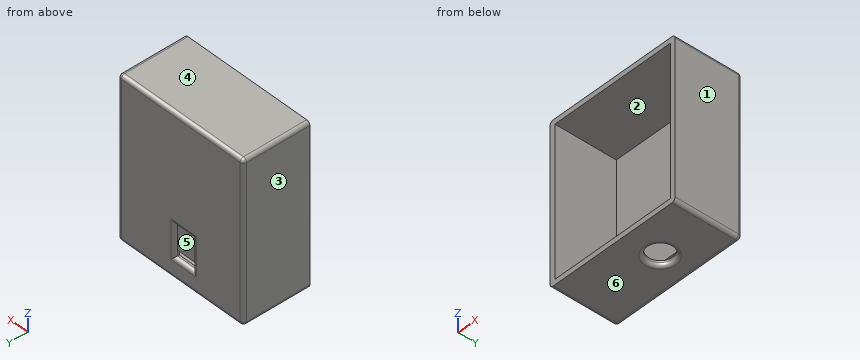
Autodesk Inventor part; units mm, degrees
ref_plane "YZ Plane" through (0, 0, 0) normal (1, 0, 0) x (0, 1, 0)
ref_plane "XZ Plane" through (0, 0, 0) normal (0, 1, 0) x (-1, 0, 0)
ref_plane "XY Plane" through (0, 0, 0) normal (0, 0, 1) x (1, 0, 0)
sketch "Sketch1" plane through (0, 0, 0) normal (0, 1, 0) x (-1, 0, 0)
  line L0 (40.3167, 41.8064) -> (-31.6833, 41.8064)
  line L1 (-31.6833, 41.8064) -> (-31.6833, -43.1936)
  line L2 (-31.6833, -43.1936) -> (40.3167, -43.1936)
  line L3 (40.3167, -43.1936) -> (40.3167, 41.8064)
  line L4 (43.3167, 44.8064) -> (-34.6833, 44.8064)
  line L5 (-34.6833, 44.8064) -> (-34.6833, -46.1936)
  line L6 (-34.6833, -46.1936) -> (43.3167, -46.1936)
  line L7 (43.3167, -46.1936) -> (43.3167, 44.8064)
  point P0 (0, 0)
  dimension "d0" = 85
  dimension "d1" = 72
  dimension "d2" = 3
  dimension "d3" = 3
  dimension "d4" = 3
  dimension "d5" = 3
extrude "Extrusion1" add sketch "Sketch1" along normal blind 35
sketch "Sketch2" plane through (0, 35, 0) normal (0, 1, 0) x (1, 0, 0)
  line L0 (34.6833, -44.8064) -> (34.6833, 46.1936)
  line L1 (-43.3167, -44.8064) -> (34.6833, -44.8064)
  line L2 (34.6833, -44.8064) -> (34.6833, 46.1936)
  line L3 (34.6833, 46.1936) -> (-43.3167, 46.1936)
  line L4 (-43.3167, 46.1936) -> (-43.3167, -44.8064)
  point P0 (0, 0)
  point P1 (34.6833, -44.8064)
extrude "Extrusion2" add sketch "Sketch2" along normal blind 3
sketch "Sketch3" plane through (34.6833, 0, 44.8064) normal (1, 0, 0) x (0, 0, -1)
  point P0 (44.8064, 0)
sketch "Sketch4" plane through (34.6833, 0, -46.1936) normal (0, 0, -1) x (-1, 0, 0)
  circle A0 centre (30.8779, 19.7188) radius 7.0099
  point P0 (34.6833, 0)
extrude "Extrusion3" cut sketch "Sketch4" against normal blind 35
sketch "Sketch5" plane through (0, 38, 0) normal (0, 1, 0) x (1, 0, 0)
  line L0 (-12.108, 16.4323) -> (-0.1673, 16.4323)
  line L1 (-0.1673, 16.4323) -> (-0.1673, 34.8019)
  line L2 (-0.1673, 34.8019) -> (-12.108, 34.8019)
  line L3 (-12.108, 34.8019) -> (-12.108, 16.4323)
  point P0 (0, 0)
extrude "Extrusion4" cut sketch "Sketch5" against normal blind 2
sketch "Sketch6" plane through (0, 36, 0) normal (0, 1, 0) x (1, 0, 0)
  point P0 (0, 0)
sketch "Sketch7" plane through (0, 36, 0) normal (0, 1, 0) x (1, 0, 0)
  line L0 (-12.108, 34.8019) -> (-0.1673, 34.8019)
  line L1 (-0.1673, 34.8019) -> (-0.1673, 16.4323)
  line L2 (-12.108, 34.8019) -> (-0.1673, 34.8019)
  line L3 (-0.1673, 34.8019) -> (-0.1673, 31.7024)
  line L4 (-0.1673, 31.7024) -> (-12.108, 31.7024)
  line L5 (-12.108, 31.7024) -> (-12.108, 34.8019)
  point P0 (0, 0)
extrude "Extrusion5" cut sketch "Sketch7" against normal blind 5
fillet "Fillet1" radius 2 10 edges at (-43.3167, 19, 44.8064) (-43.3167, 19, -46.1936) (-4.3167, 38, -46.1936) (-43.3167, 38, -0.6936) (34.6833, 38, -0.6936) (-6.1377, 38, -16.4323) (-0.1673, 38, -25.6171) (-12.108, 38, -25.6171) (-6.1377, 38, -34.8019) (-4.3167, 38, 44.8064)
fillet "Fillet2" radius 2 4 edges at (34.0975, 37.4142, 44.2206) (34.6833, 18.0001, 44.8064) (34.0975, 37.4142, -45.6079) (34.6833, 18.0001, -46.1936)
fillet "Fillet3" radius 2 1 edges at (10.8153, 19.7188, -46.1936)
properties part number "198MainChassis"
Here's how the part is built. I have some questions about the finished solid (model axes, mm). Face numbers are marked on the shaded views. A direction names the side the tool comes from. Coordinates: 2 decimals unless noted, no trailing zeros. Write each loop counter-clockwise with the first axis right and the second up, starting at its lowest first coordinate (ties: lowest second). Pieces come first, ordered by that corner, then holes. Notation, with made-up numbers: (81.5, -38) - (132.5, -38) arc R25 cw to (132.5, -24) - close; hole circle Ø3 at (86, 29). An arc over 180 degrees is marked (long way). Use one line per item in the form item = value.
1) Suppose I cut it at B-B, the plane y = 31. Write out the boundary of the cut face in (x, z), plus the area to 3 significant figures.
Solved:
outline = (-43.32, -44.19) arc R2 ccw to (-41.32, -46.19) - (32.68, -46.19) arc R2 ccw to (34.68, -44.19) - (34.68, 42.81) arc R2 ccw to (32.68, 44.81) - (-41.32, 44.81) arc R2 ccw to (-43.32, 42.81) - close; hole (-40.32, -43.19) - (31.68, -43.19) - (31.68, 41.81) - (-40.32, 41.81) - close
area = 975 mm2
2) I need wall thicknesses on line 1 (Z direction, x = -24, y = 12.5); line 2 (X direction, y = 24, z = 22); line 3 (Y direction, x = 20, z = -18). Which ranges of each line are inside material? Lowest first, please.
Solved:
line_1 = -46.19 to -43.19, 41.81 to 44.81
line_2 = -43.32 to -40.32, 31.68 to 34.68
line_3 = 35 to 38
3) Suppose I cut it at D-D, the plane x = 25. Write out the boundary of the cut face in (y, z).
Solved:
outline = (0, -46.19) - (36, -46.19) arc R2 ccw to (38, -44.19) - (38, 42.81) arc R2 ccw to (36, 44.81) - (0, 44.81) - (0, 41.81) - (35, 41.81) - (35, -43.19) - (0, -43.19) - close
4) Suppose I cut it at C-C, the plane z = -40. Write out the boundary of the cut face in (x, y), plus the area to 3 significant figures.
Solved:
outline = (-43.32, 0) - (-40.32, 0) - (-40.32, 35) - (31.68, 35) - (31.68, 0) - (34.68, 0) - (34.68, 36) arc R2 ccw to (32.68, 38) - (-41.32, 38) arc R2 ccw to (-43.32, 36) - close
area = 442 mm2
5) On a 3-axis mill with a long thin cutter (end or side, diameter ignored), from which of +Z, -Z, +X, -X, +Y, -Y can I reach the whole of each face in a straight line? I mean the marked faces 1 and 2. Say none if no direction works.
Solved:
face_1 = +Z, -Z, +X, +Y, -Y
face_2 = -Y
6) I'm going to push flat-ended pins straight in: P1, Ø11, axis at x = 3.81, y = 19.72, coming from the -Z side; P2, Ø9.5, axis at x = -6, z = -26.5, coming from the +Y side; P3, Ø2, axis at x = -10.5, z = -3, coming from the -Y side. Where does each tip first touch, or does it pass through?
Solved:
P1 = 41.81
P2 = 36
P3 = 35
7) Thinking about a two-plate mould opening in Z: for the marked faces 3, 4, 5 and 6, which applies, released by +Z, released by -Z, zero draft, split by the parting line, or undercut?
Solved:
face_3 = zero draft
face_4 = released by +Z
face_5 = undercut
face_6 = released by -Z
